For this review, take the finished solid that the model builds, in its own axes (mm). Round coordinates to 2 decimals unless told otherwise and drop trailing zeros. Write each loop counter-clockwise with the first axis right and the second up, starting at its lowest first coordinate (ties: lowest second). Pieces come first, ordered by that corner, then holes.
from build123d import *

# Parameters (mm, degrees)
F1_DEPTH = 76.2
F2_DEPTH = 6.35
F3_R     = 5.08


# Not quite as in the source:
# - the program builds the solid bodies; features that only make, move or delete a surface that nothing else refers to are left out


with BuildPart() as f1:
    # F0 (on Front) → F1 (new body, symmetric)
    with BuildSketch(Plane.XZ):
        Polygon((34.29, -3.175), (38.1, -3.175), (38.1, 3.175), (-38.1, 3.175), (-38.1, -3.175), (-34.29, -3.175), align=None)
    extrude(amount=F1_DEPTH, both=True)

    # F0 (on Front) → F2 (join)
    with BuildSketch(Plane.XZ):
        Polygon((34.29, -3.175), (38.1, -3.175), (38.1, 3.175), (-38.1, 3.175), (-38.1, -3.175), (-34.29, -3.175), align=None)
    extrude(amount=F2_DEPTH)

    # F3
    f3_edges = [f1.edges().sort_by_distance(p)[0] for p in [
        (38.1, 0, -3.175),
        (0, -76.2, -3.175),
        (-38.1, 0, -3.175),
        (0, 76.2, -3.175),
    ]]
    fillet(f3_edges, radius=F3_R)


solid = f1.part
(1) For line 1 along X through (y, z) = (-61, 1.75); line 2 along Y through (x, z) = (0, 1.5); line 3 along X through (y, z) = (-57.5, -2), list the stretches that pass through material, from the lowest coordinate up.
Geometry check:
line 1: x = -38.1 to 38.1
line 2: y = -76.18 to 76.18
line 3: x = -36.27 to 36.27
(2) We need section A-A, the plane y = -41. Give the boundary of the cut face in (x, z) (3 decimals).
Geometry check:
outline: (-38.1, 1.905) arc R5.08 ccw to (-33.02, -3.175) - (33.02, -3.175) arc R5.08 ccw to (38.1, 1.905) - (38.1, 3.175) - (-38.1, 3.175) - close
(3) For pin 1 Ø1 at (y, z) = (-2, -2) entering from +X, flat-tipped, find the tip position at first contact; note if it passes through.
Geometry check:
pin 1: stops at x = 36.79
(4) We need section B-B, the plane z = -0.5. Give the boundary of the cut face in (x, y), and give its area (3 significant figures).
Geometry check:
outline: (-37.49, -75.59) - (37.49, -75.59) - (37.49, 75.59) - (-37.49, 75.59) - close
area: 11,300 mm2
